```python
from build123d import *

# Parameters (mm, degrees)
SKETCH1_W               = 8
SKETCH1_H               = 8
BOSS_EXTRUDE1_DEPTH     = 3
CUT_EXTRUDE1_DEPTH      = 12.704699911
CUT_EXTRUDE1_DEPTH_BACK = 12.704699911
CUT_EXTRUDE2_DEPTH      = 11
SKETCH4_R               = 1.75
CUT_EXTRUDE3_DEPTH      = 0.4
SKETCH5_W               = 8
SKETCH5_H               = 1
BOSS_EXTRUDE2_DEPTH     = 2
FILLET1_R               = 4
SKETCH6_W               = 2.10217216
SKETCH6_H               = 1.6
CUT_EXTRUDE4_DEPTH      = 0.4


with BuildPart() as part:
    # Sketch1 → Boss-Extrude1 (new body)
    with BuildSketch(Plane(origin=(0, 0, 0), x_dir=(1, 0, 0), z_dir=(0, 1, 0))):
        with Locations((4, 4)):
            Rectangle(SKETCH1_W, SKETCH1_H)
    extrude(amount=BOSS_EXTRUDE1_DEPTH)

    # Sketch2 → Cut-Extrude1 (cut, two sides: drawn at the far end of the back side and taken through both)
    with BuildSketch(Plane.XY.offset(-CUT_EXTRUDE1_DEPTH_BACK)):
        Polygon((0, 0), (0.6, 3), (0, 3), align=None)
        Polygon((8, 0), (7.4, 3), (8, 3), align=None)
    extrude(amount=CUT_EXTRUDE1_DEPTH + CUT_EXTRUDE1_DEPTH_BACK, mode=Mode.SUBTRACT)

    # Sketch3 → Cut-Extrude2 (cut)
    with BuildSketch(Plane(origin=(0, 0, 0), x_dir=(0, 0, -1), z_dir=(1, 0, 0))):
        Polygon((0, 0), (0.6, 3), (0, 3), align=None)
        Polygon((8, 3), (7.4, 3), (8, 0), align=None)
    extrude(amount=CUT_EXTRUDE2_DEPTH, mode=Mode.SUBTRACT)

    # Sketch4 → Cut-Extrude3 (cut)
    with BuildSketch(Plane.XZ):
        with Locations(Location((4, -3.75, 0), (0, 0, 270))):
            Circle(SKETCH4_R)
    extrude(amount=-CUT_EXTRUDE3_DEPTH, mode=Mode.SUBTRACT)

    # Sketch5 → Boss-Extrude2 (add)
    with BuildSketch(Plane.XZ):
        with Locations((4, -7.5)):
            Rectangle(SKETCH5_W, SKETCH5_H)
    extrude(amount=BOSS_EXTRUDE2_DEPTH)

    # Fillet1
    # the kernel refuses this fillet: 4 mm, written as the material it takes off along each edge
    with BuildSketch(Plane(origin=(8, -2, -16.660254038), x_dir=(0, 1, 0), z_dir=(0, 0, 1)), Plane(origin=(0, -2, 1.660254038), x_dir=(0, 1, 0), z_dir=(0, 0, -1))) as fillet1_piece_1:
        with BuildLine():
            CenterArc((4, 3.464101615), FILLET1_R, 180, 60)
            Line((0, 3.464101615), (-0.08, 3.464101615))
            Line((-0.08, 3.464101615), (-0.08, 0))
            Line((-0.08, 0), (0, -0.08))
            ThreePointArc((0, -0.08), (1, -0.08), (1.96, -0.069282032))
            Line((1.96, -0.069282032), (2, 0))
        make_face()
    extrude(amount=18.320508076, mode=Mode.SUBTRACT)

    # Sketch6 → Cut-Extrude4 (cut)
    with BuildSketch(Plane(origin=(0, 3, 0), x_dir=(1, 0, 0), z_dir=(0, 1, 0))):
        Polygon((3.09782784, 2.1), (3.09782784, 3.7), (3.09782784, 4.7), (1.1, 2.9), (3.09782784, 1.1), align=None)
        with Locations((4.14891392, 2.9)):
            Rectangle(SKETCH6_W, SKETCH6_H)
        Polygon((5.2, 6.8), (5.2, 3.7), (5.2, 2.1), (6.8, 2.1), (6.8, 6.8), align=None)
    extrude(amount=-CUT_EXTRUDE4_DEPTH, mode=Mode.SUBTRACT)


solid = part.part
```
Part model, mm, in its own coordinate system. A direction names the side the tool comes from. Round coordinates to 2 decimals unless told otherwise and drop trailing zeros. Write each loop counter-clockwise with the first axis right and the second up, starting at its lowest first coordinate (ties: lowest second). Pieces come first, ordered by that corner, then holes.
Item 1: Drop flat-ended pins along their axis: pin 1 Ø3 at (x, z) = (5, -3.5) entering from -Y; pin 2 Ø2 at (x, y) = (3, -1.5) entering from +Z; pin 3 Ø1.8 at (x, z) = (3.5, -3.5) entering from -Y. Give the stop position or say it passes through.
Results:
pin 1: stops at y = 0
pin 2: stops at z = -7
pin 3: stops at y = 0.4
Item 2: Which spindle directions (+Z, -Z, +X, -X, +Y, -Y) get a long thin tool onto all of the face, cutting with end or side? Do faces 5 (the flat face through (2.1, 2.8, -2)), 6 (the flat face through (4, 0.4, -4)), 7 (the flat face through (4, -1, -7)), 8 (the flat face through (3.9, 1.5, -7.7)), 9 (the cylindrical face through (6.51, -1.48, -7.51)). Say none if no direction does.
Results:
face 5: +Y
face 6: -Y
face 7: +Z, +X, -X, -Y
face 8: -Z, +X, -X, +Y
face 9: +Z, -Z, +X, -Y
Item 3: Cut at A-A, the plane x = 4. Give the cut face in (y, z).
Results:
outline: (-2, -8) - (0, -8) - (3, -7.4) - (3, -3.7) - (2.6, -3.7) - (2.6, -2.1) - (3, -2.1) - (3, -0.6) - (0, 0) - (0, -2) - (0.4, -2) - (0.4, -5.5) - (0, -5.5) - (0, -7) - (-2, -7) - close
Item 4: Two-plate mould, pull along Z, no slides. Class faces 1 (the flat face through (3.9, 1.5, -0.3)), 2 (the cylindrical face through (2.94, 0.2, -2.36)), 3 (the flat face through (0.3, 1.5, -4.1)), 4 (the flat face through (2.1, 2.8, -3.8)): +Z half, -Z half, draft (parallel to the pull), parting line (faces both ways), or undercut.
Results:
face 1: +Z half
face 2: undercut
face 3: draft
face 4: undercut
Item 5: Probe L1, parallel to Y at x = 6.75, z = -1.5; L2, parallel to Y at x = 6.75, z = -3.75; L3, parallel to X at y = 0.35, z = -3.75. List the from-to ranges inside material, lowest first.
Results:
L1: y = 0 to 3
L2: y = 0 to 2.6
L3: x = 0.07 to 2.25, 5.75 to 7.93
Item 6: Cut at C-C, the plane y = 1.45. Give the cut face in (x, z), plus the area to 3 significant figures.
Results:
outline: (0.29, -7.71) - (7.71, -7.71) - (7.71, -0.29) - (0.29, -0.29) - close
area: 55.1 mm2
Item 7: Cut at B-B, the plane z = -6.5. Give the cut face in (x, y).
Results:
outline: (0, 0) - (8, 0) - (7.4, 3) - (6.8, 3) - (6.8, 2.6) - (5.2, 2.6) - (5.2, 3) - (0.6, 3) - close
Item 8: Cut at D-D, the plane z = -1. Give the cut face in (x, y), plus the area to 3 significant figures.
Results:
outline: (0, 0) - (8, 0) - (7.4, 3) - (0.6, 3) - close
area: 22.2 mm2
